```python
from build123d import *

# Parameters (mm, degrees)
F0_W     = 152.5
F0_H     = 152.5
F0_R     = 13.25
F1_DEPTH = 1
F2_DEPTH = 2
F3_R     = 2.55
F4_DEPTH = 2.001


with BuildPart() as f1:
    # F0 (on Top) → F1 (new body)
    with BuildSketch(Plane.XY):
        Rectangle(F0_W, F0_H)
        with Locations((-60, -60)):
            Circle(F0_R, mode=Mode.SUBTRACT)
        with Locations((-30, -60)):
            Circle(F0_R, mode=Mode.SUBTRACT)
        with Locations((-60, -30)):
            Circle(F0_R, mode=Mode.SUBTRACT)
        with Locations((-30, -30)):
            Circle(F0_R, mode=Mode.SUBTRACT)
        with Locations((0, -60)):
            Circle(F0_R, mode=Mode.SUBTRACT)
        with Locations((30, -60)):
            Circle(F0_R, mode=Mode.SUBTRACT)
        with Locations((60, -60)):
            Circle(F0_R, mode=Mode.SUBTRACT)
        with Locations((0, -30)):
            Circle(F0_R, mode=Mode.SUBTRACT)
        with Locations((30, -30)):
            Circle(F0_R, mode=Mode.SUBTRACT)
        with Locations((60, -30)):
            Circle(F0_R, mode=Mode.SUBTRACT)
        with Locations((-60, 0)):
            Circle(F0_R, mode=Mode.SUBTRACT)
        with Locations((-60, 30)):
            Circle(F0_R, mode=Mode.SUBTRACT)
        with Locations((-30, 0)):
            Circle(F0_R, mode=Mode.SUBTRACT)
        with Locations((-30, 30)):
            Circle(F0_R, mode=Mode.SUBTRACT)
        with Locations((-60, 60)):
            Circle(F0_R, mode=Mode.SUBTRACT)
        with Locations((-30, 60)):
            Circle(F0_R, mode=Mode.SUBTRACT)
        Circle(F0_R, mode=Mode.SUBTRACT)
        with Locations((30, 0)):
            Circle(F0_R, mode=Mode.SUBTRACT)
        with Locations((0, 30)):
            Circle(F0_R, mode=Mode.SUBTRACT)
        with Locations((30, 30)):
            Circle(F0_R, mode=Mode.SUBTRACT)
        with Locations((60, 0)):
            Circle(F0_R, mode=Mode.SUBTRACT)
        with Locations((60, 30)):
            Circle(F0_R, mode=Mode.SUBTRACT)
        with Locations((0, 60)):
            Circle(F0_R, mode=Mode.SUBTRACT)
        with Locations((30, 60)):
            Circle(F0_R, mode=Mode.SUBTRACT)
        with Locations((60, 60)):
            Circle(F0_R, mode=Mode.SUBTRACT)
        with Locations((-60, 60)):
            Circle(F0_R)
        with Locations((-30, 60)):
            Circle(F0_R)
        with Locations((0, 60)):
            Circle(F0_R)
        with Locations((30, 60)):
            Circle(F0_R)
        with Locations((60, 60)):
            Circle(F0_R)
        with Locations((60, 30)):
            Circle(F0_R)
        with Locations((30, 30)):
            Circle(F0_R)
        with Locations((-30, 30)):
            Circle(F0_R)
        with Locations((-60, 30)):
            Circle(F0_R)
        with Locations((0, 30)):
            Circle(F0_R)
        Circle(F0_R)
        with Locations((-30, 0)):
            Circle(F0_R)
        with Locations((-60, 0)):
            Circle(F0_R)
        with Locations((30, 0)):
            Circle(F0_R)
        with Locations((60, 0)):
            Circle(F0_R)
        with Locations((30, -30)):
            Circle(F0_R)
        with Locations((60, -30)):
            Circle(F0_R)
        with Locations((60, -60)):
            Circle(F0_R)
        with Locations((30, -60)):
            Circle(F0_R)
        with Locations((0, -60)):
            Circle(F0_R)
        with Locations((0, -30)):
            Circle(F0_R)
        with Locations((-30, -60)):
            Circle(F0_R)
        with Locations((-30, -30)):
            Circle(F0_R)
        with Locations((-60, -30)):
            Circle(F0_R)
        with Locations((-60, -60)):
            Circle(F0_R)
    extrude(amount=F1_DEPTH)

    # F0 (on Top) → F2 (join)
    with BuildSketch(Plane.XY):
        Rectangle(F0_W, F0_H)
        with Locations((-60, -60)):
            Circle(F0_R, mode=Mode.SUBTRACT)
        with Locations((-30, -60)):
            Circle(F0_R, mode=Mode.SUBTRACT)
        with Locations((-60, -30)):
            Circle(F0_R, mode=Mode.SUBTRACT)
        with Locations((-30, -30)):
            Circle(F0_R, mode=Mode.SUBTRACT)
        with Locations((0, -60)):
            Circle(F0_R, mode=Mode.SUBTRACT)
        with Locations((30, -60)):
            Circle(F0_R, mode=Mode.SUBTRACT)
        with Locations((60, -60)):
            Circle(F0_R, mode=Mode.SUBTRACT)
        with Locations((0, -30)):
            Circle(F0_R, mode=Mode.SUBTRACT)
        with Locations((30, -30)):
            Circle(F0_R, mode=Mode.SUBTRACT)
        with Locations((60, -30)):
            Circle(F0_R, mode=Mode.SUBTRACT)
        with Locations((-60, 0)):
            Circle(F0_R, mode=Mode.SUBTRACT)
        with Locations((-60, 30)):
            Circle(F0_R, mode=Mode.SUBTRACT)
        with Locations((-30, 0)):
            Circle(F0_R, mode=Mode.SUBTRACT)
        with Locations((-30, 30)):
            Circle(F0_R, mode=Mode.SUBTRACT)
        with Locations((-60, 60)):
            Circle(F0_R, mode=Mode.SUBTRACT)
        with Locations((-30, 60)):
            Circle(F0_R, mode=Mode.SUBTRACT)
        Circle(F0_R, mode=Mode.SUBTRACT)
        with Locations((30, 0)):
            Circle(F0_R, mode=Mode.SUBTRACT)
        with Locations((0, 30)):
            Circle(F0_R, mode=Mode.SUBTRACT)
        with Locations((30, 30)):
            Circle(F0_R, mode=Mode.SUBTRACT)
        with Locations((60, 0)):
            Circle(F0_R, mode=Mode.SUBTRACT)
        with Locations((60, 30)):
            Circle(F0_R, mode=Mode.SUBTRACT)
        with Locations((0, 60)):
            Circle(F0_R, mode=Mode.SUBTRACT)
        with Locations((30, 60)):
            Circle(F0_R, mode=Mode.SUBTRACT)
        with Locations((60, 60)):
            Circle(F0_R, mode=Mode.SUBTRACT)
    extrude(amount=F2_DEPTH)

    # F3 (on face) → F4 (cut, through all)
    with BuildSketch(Plane.XY.offset(2)):
        with Locations((-72.2, 72.2)):
            Circle(F3_R)
        with Locations((72.2, 72.2)):
            Circle(F3_R)
        with Locations((45, 15)):
            Circle(F3_R)
        with Locations((-45, 15)):
            Circle(F3_R)
        with Locations((45, -15)):
            Circle(F3_R)
        with Locations((-45, -15)):
            Circle(F3_R)
        with Locations((-72.2, -72.2)):
            Circle(F3_R)
        with Locations((72.2, -72.2)):
            Circle(F3_R)
    extrude(amount=-F4_DEPTH, mode=Mode.SUBTRACT)


solid = f1.part
```
Build history of the part. All positions in model axes, mm. A direction names the side the tool comes from. Round coordinates to 2 decimals unless told otherwise and drop trailing zeros. Loops run counter-clockwise (first coordinate to the right, second up) from the corner with the lowest first, then second, coordinate; pieces in that order, holes last.
Item 1: Pin check, flat tips, straight feed: P1, Ø21, axis at x = 29.5, y = 32.5, coming from the +Z side; P2, Ø12, axis at x = -38, y = 59.5, coming from the +Z side. Stop position of each tip, or through.
Item 2: Saw through at D-D (x = -39). List the corners of the cut face in (y, z), then the cut area to 3 significant figures.
Item 3: Saw through at A-A (y = -15). List the corners of the cut face in (x, z), then the cut area to 3 significant figures.
Item 4: Saw through at B-B (x = 45). List the corners of the cut face in (y, z).
Item 5: Saw through at C-C (y = -60). List the corners of the cut face in (x, z), then the cut area to 4 significant figures.
Item 6: Which spindle directions (+Z, -Z, +X, -X, +Y, -Y) get a long thin tool onto all of the face, cutting with end or side? Do faces 1 (the face through (42.452, 15.112, 1.014)), 2 (the face through (30, 30, 1)). Say none if no direction does.
Item 7: Drill centre lines: line 1 along Y through (x, z) = (30, 1.6); line 2 along X through (y, z) = (-29.5, 1.5); line 3 along Y through (x, z) = (72.2, 0.7). Where is each one in solid material? Low to high.
Worked answers:
1. P1: stops at z = 1
1. P2: stops at z = 2
2. outline: (-76.25, 0) - (76.25, 0) - (76.25, 2) - (69.72, 2) - (69.72, 1) - (50.28, 1) - (50.28, 2) - (39.72, 2) - (39.72, 1) - (20.28, 1) - (20.28, 2) - (9.72, 2) - (9.72, 1) - (-9.72, 1) - (-9.72, 2) - (-20.28, 2) - (-20.28, 1) - (-39.72, 1) - (-39.72, 2) - (-50.28, 2) - (-50.28, 1) - (-69.72, 1) - (-69.72, 2) - (-76.25, 2) - close
2. area: 208 mm2
3. outline: (-76.25, 0) - (-47.55, 0) - (-47.55, 2) - (-76.25, 2) - close; (-42.45, 0) - (42.45, 0) - (42.45, 2) - (-42.45, 2) - close; (47.55, 0) - (76.25, 0) - (76.25, 2) - (47.55, 2) - close
3. area: 285 mm2
4. outline: (-76.25, 0) - (-17.55, 0) - (-17.55, 2) - (-76.25, 2) - close; (-12.45, 0) - (12.45, 0) - (12.45, 2) - (-12.45, 2) - close; (17.55, 0) - (76.25, 0) - (76.25, 2) - (17.55, 2) - close
5. outline: (-76.25, 0) - (76.25, 0) - (76.25, 2) - (73.25, 2) - (73.25, 1) - (46.75, 1) - (46.75, 2) - (43.25, 2) - (43.25, 1) - (16.75, 1) - (16.75, 2) - (13.25, 2) - (13.25, 1) - (-13.25, 1) - (-13.25, 2) - (-16.75, 2) - (-16.75, 1) - (-43.25, 1) - (-43.25, 2) - (-46.75, 2) - (-46.75, 1) - (-73.25, 1) - (-73.25, 2) - (-76.25, 2) - close
5. area: 172.5 mm2
6. face 1: +Z, -Z
6. face 2: +Z
7. line 1: y = -76.25 to -73.25, -46.75 to -43.25, -16.75 to -13.25, 13.25 to 16.75, 43.25 to 46.75, 73.25 to 76.25
7. line 2: x = -76.25 to -73.24, -46.76 to -43.24, -16.76 to -13.24, 13.24 to 16.76, 43.24 to 46.76, 73.24 to 76.25
7. line 3: y = -76.25 to -74.75, -69.65 to 69.65, 74.75 to 76.25
